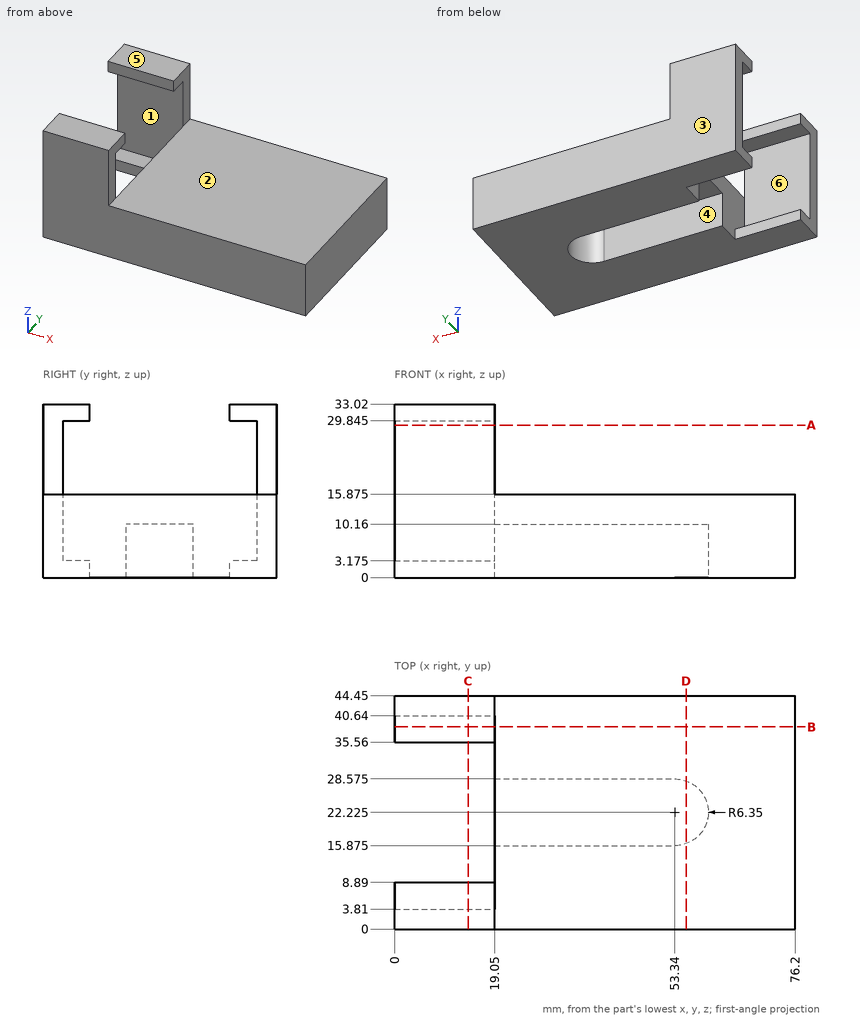
Geometry: see drawing. Coordinates: mm, zero at the bounding-box minimum. A direction names the side the tool comes from. Give positions to 0.01 mm unless a question says otherwise; leave off trailing zeros. Order: outer loops, then holes, each group sorted by start corner. A loop starts at its lowest first (then second) coordinate and runs counter-clockwise, first axis right, second up. Notation, with made-up numbers: (-12.5, 89.25) -> (11.5, 89.25) arc R30 cw to (11.5, 117.25) -> close; hole circle Ø2 at (64, 7.5). An arc over 180 degrees is marked (long way). Write each question's results on one line, items separated by ' | '. Start each with the question number.
1) Section B-B (y = 38.5). Return loops of the section in (x, z) (3 decimals), then the cut area to 3 significant figures.
2) Section C-C (x = 14). Return loops of the section in (y, z) (3 decimals).
3) Draft query along Z for the marked faces 1, 2 and 3. Return one class per face: pulls with the +Z half, pulls with the -Z half, needs draft (parallel to the pull), parting line crosses it, or undercut.
4) First-contact query: pin 1 (4.5 mm diameter, centred on y = 3, z = 24.5, fed in from +X); pin 2 (1.5 mm diameter, centred on y = 7.5, z = 4.5, fed in from -X); pin 3 (6.5 mm diameter, centred on x = 32.5, y = 20, fed in from -Z). Flat tips, straight axial feed; report the tip coordinate or a pass-through.
5) Section D-D (x = 55.5). Return loops of the section in (y, z) (3 decimals), then the cut area to 3 significant figures.
6) Line query: line 1 (Y direction, x = 17.5, z = 26); line 2 (Z direction, x = 46.5, y = 5.5) (3 decimals); line 3 (Z direction, x = 39.5, y = 17) (3 decimals). Output: solid intervals per line, ascending. Write a range as from..to.
7) Section A-A (z = 29). Return loops of the section in (x, y).
8) Set-up query: the marked faces 4, 5 and 6. Return all of +Z, -Z, +X, -X, +Y, -Y with unobstructed straight access to the full face (end or side cutting, diameter ignored); none if empty.
Calculated:
1) outline: (0, 0) -> (76.2, 0) -> (76.2, 15.875) -> (19.05, 15.875) -> (19.05, 3.175) -> (0, 3.175) -> close; (0, 29.845) -> (19.05, 29.845) -> (19.05, 33.02) -> (0, 33.02) -> close | area: 1,030 mm2
2) outline: (0, 0) -> (8.89, 0) -> (8.89, 3.175) -> (3.81, 3.175) -> (3.81, 29.845) -> (8.89, 29.845) -> (8.89, 33.02) -> (0, 33.02) -> close; (35.56, 0) -> (44.45, 0) -> (44.45, 33.02) -> (35.56, 33.02) -> (35.56, 29.845) -> (40.64, 29.845) -> (40.64, 3.175) -> (35.56, 3.175) -> close
3) face 1: undercut | face 2: pulls with the +Z half | face 3: needs draft
4) pin 1: x = 19.05 | pin 2: x = 19.05 | pin 3: z = 10.16
5) outline: (0, 0) -> (16.254, 0) -> (16.254, 10.16) -> (28.196, 10.16) -> (28.196, 0) -> (44.45, 0) -> (44.45, 15.875) -> (0, 15.875) -> close | area: 584 mm2
6) line 1: 0..3.81, 40.64..44.45 | line 2: 0..15.875 | line 3: 10.16..15.875
7) outline: (0, 0) -> (19.05, 0) -> (19.05, 3.81) -> (0, 3.81) -> close; (0, 40.64) -> (19.05, 40.64) -> (19.05, 44.45) -> (0, 44.45) -> close
8) face 4: -Z, -X | face 5: +Z, +X, -X, +Y, -Y | face 6: -X
